Work out the finished part from the listing and answer in its coordinate system (mm). A direction names the side the tool comes from. Coordinates: 2 decimals unless noted, no trailing zeros. Order: outer loops, then holes, each group sorted by start corner. A loop starts at its lowest first (then second) coordinate and runs counter-clockwise, first axis right, second up. Notation, with made-up numbers: (16.25, 17) - (51.25, 17) arc R30 cw to (51.25, 42) - close; hole circle Ø3 at (75, -14). An arc over 180 degrees is marked (long way). Answer as a JSON object with one key per item and string values. Group by question number.
1) Section D-D (z = 10.25) is taken. Give the vertices of the cut face in (x, y), plus the area to 3 significant figures.
2) A tool of negligible diameter and unlimited length cuts with its end or side. For faces 1 (the face through (-1.437, 1.318, 9.423)), 2 (the face through (-1.08, -4.88, 7.17)), from which of +Z, -Z, +X, -X, +Y, -Y can it reach the whole face along a straight path? Write none if from no direction.
3) Section C-C (z = 2.25) is taken. Give the vertices of the cut face in (x, y), plus the area to 3 significant figures.
4) Find the intervals of material crossed by line 1 along Y through (x, z) = (0, -3.5); line 2 along Y through (x, z) = (0, 11.5); line 3 along X through (y, z) = (-0.25, -6), in increasing order.
5) The mould has two halves that part along X. Classify faces 3 (the face through (3.233, -1.341, -2.084)), 4 (the face through (2, -2, 4)), 5 (the face through (-6, 0, -3)), 6 (the face through (2.2, -3.3, -8)): released by +X, released by -X, zero draft, split by the parting line, or undercut.
6) Each of these flat-tipped pins is pushed along its axis until it touches: P1, Ø1, axis at x = -4, y = 4, coming from the +Z side; P2, Ø4.5, axis at x = 0, y = 0, coming from the +Z side; P3, Ø6, axis at x = -1.5, z = 12, coming from the -Y side; P4, Ø1, axis at x = -1.5, z = -3, coming from the +Y side. Where does it stop, or does it pass through?
7) Section A-A (y = 0) is taken. Give the vertices of the cut face in (x, z), plus the area to 3 significant figures.
from build123d import *

# Parameters (mm, degrees)
SKETCH_1_R          = 5
SKETCH_1_R_2        = 1.95
EXTRUDE_1_DEPTH     = 15
SKETCH_3_R          = 3.5
CUT_EXTRUDE_1_DEPTH = 4
EXTRUDE_START       = -8
SKETCH_4_R          = 6
SKETCH_4_R_2        = 3.5
EXTRUDE_2_DEPTH     = 8
CHAMFER_1_SIZE      = 1.5
CHAMFER_2_SIZE      = 1
CUT_EXTRUDE_START   = -2
SKETCH_9_R          = 5
SKETCH_9_R_2        = 4.2
CUT_EXTRUDE_4_DEPTH = 2


with BuildPart() as part:
    # 스케치1 → 보스-돌출1 (new body)
    with BuildSketch(Plane.XY):
        Circle(SKETCH_1_R)
        Circle(SKETCH_1_R_2, mode=Mode.SUBTRACT)
    extrude(amount=EXTRUDE_1_DEPTH)

    # 스케치3 → 컷-돌출1 (cut)
    with BuildSketch(Plane.XY):
        Circle(SKETCH_3_R)
    extrude(amount=CUT_EXTRUDE_1_DEPTH, mode=Mode.SUBTRACT)

    # 스케치4 → 보스-돌출2 (add)
    with BuildSketch(Plane.XY.offset(EXTRUDE_START)):
        Circle(SKETCH_4_R)
        Circle(SKETCH_4_R_2, mode=Mode.SUBTRACT)
    extrude(amount=EXTRUDE_2_DEPTH)

    # 모따기1
    # the kernel refuses this chamfer: 1.5 mm, written as the material it adds along each edge
    with BuildSketch(Plane(origin=(0, 0, 0), x_dir=(1, 0, 0), z_dir=(0, -1, 0))) as chamfer_1_piece_1_section:
        Polygon((5, CHAMFER_1_SIZE), (5 + CHAMFER_1_SIZE, 0), (5, 0), align=None)
    chamfer_1_piece_1 = revolve(axis=Axis((0, 0, 0), (0, 0, 1)), mode=Mode.PRIVATE)
    chamfer_1_piece_1 = chamfer_1_piece_1 & Plane(origin=(0, 0, 0.997696527), x_dir=(1, 0, 0), z_dir=(0, 0, -1)) * Cylinder(6, 26, mode=Mode.PRIVATE)
    add(chamfer_1_piece_1)

    # 모따기2
    chamfer_2_edges = [part.edges().sort_by_distance(p)[0] for p in [
        (-6, 0, -8),
    ]]
    chamfer(chamfer_2_edges, length=CHAMFER_2_SIZE)

    # 스케치9 → 컷-돌출4 (cut)
    with BuildSketch(Plane.XY.offset(15).offset(CUT_EXTRUDE_START)):
        Circle(SKETCH_9_R)
        Circle(SKETCH_9_R_2, mode=Mode.SUBTRACT)
    extrude(amount=CUT_EXTRUDE_4_DEPTH, mode=Mode.SUBTRACT)


solid = part.part
Report:
{
 "1": {"outline": "circle Ø10 at (0, 0); hole circle Ø3.9 at (0, 0)", "area": "66.6 mm²"},
 "2": {"face 1": "+Z, -Z", "face 2": "+Z"},
 "3": {"outline": "circle Ø10 at (0, 0); hole circle Ø7 at (0, 0)", "area": "40.1 mm²"},
 "4": {"line 1": "y = -6 to -3.5, 3.5 to 6", "line 2": "y = -5 to -1.95, 1.95 to 5", "line 3": "x = -5.99 to -3.49, 3.49 to 5.99"},
 "5": {"face 3": "undercut", "face 4": "undercut", "face 5": "split by the parting line", "face 6": "zero draft"},
 "6": {"P1": "stops at z = 1.34", "P2": "stops at z = 15", "P3": "stops at y = -5", "P4": "stops at y = 5.92"},
 "7": {"outline": "(-6, -7) - (-5, -8) - (-3.5, -8) - (-3.5, 4) - (-1.95, 4) - (-1.95, 15) - (-4.2, 15) - (-4.2, 13) - (-5, 13) - (-5, 1.5) - (-6, 0.5) - close; (1.95, 4) - (3.5, 4) - (3.5, -8) - (5, -8) - (6, -7) - (6, 0.5) - (5, 1.5) - (5, 13) - (4.2, 13) - (4.2, 15) - (1.95, 15) - close", "area": "117 mm²"}
}
